Part print with two shaded views. Sizes in mm from the minimum x, y, z corner. A direction names the side the tool comes from. Round coordinates to 2 decimals unless told otherwise and drop trailing zeros. Write each loop counter-clockwise with the first axis right and the second up, starting at its lowest first coordinate (ties: lowest second). Pieces come first, ordered by that corner, then holes. Notation, with made-up numbers: M 74,49 L 110,49 A16 cw 110,74 Z; hole C 47,85.5 d4. An arc over 180 degrees is marked long. Use one line per item in the form item = value. Start each with the question number.
Item 1: Cut at C-C, the plane y = 4.75. Give the cut face in (x, z) (1 decimal).
Item 2: Flat gauge pins, fed straight in: pin 1 Ø1 at (y, z) = (1.5, 16) entering from +X; pin 2 Ø4 at (x, z) = (31.51, 12.7) entering from -Y; pin 3 Ø1.8 at (x, z) = (12.46, 12.7) entering from +Y; pin 4 Ø1.5 at (x, y) = (6, 3) entering from -Z. Where does each tip first touch, or does it go through?
Item 3: Mould opens along Z. For the marked faces 1, 2, 3 and 4 say: +Z half, -Z half, draft (parallel to the pull), parting line (faces both ways), or undercut.
Item 4: Probe L1, parallel to X at y = 4.5, z = 12.7 (1 decimal); L2, parallel to X at y = 3.75, z = 10 (1 decimal); L3, parallel to Y at x = 29, z = 9.5. List the from-to ranges inside material, lowest first.
Item 5: Which spindle directions (+Z, -Z, +X, -X, +Y, -Y) get a long thin tool onto all of the face, cutting with end or side? Do the marked faces 5, 6 and 7. Say none if no direction does.
Item 6: Cut at A-A, the plane z = 12.7. Give the cut face in (x, y) (1 decimal).
Item 7: Cut at B-B, the plane x = 32. Give the cut face in (y, z) (1 decimal), then the cut area to 3 significant figures.
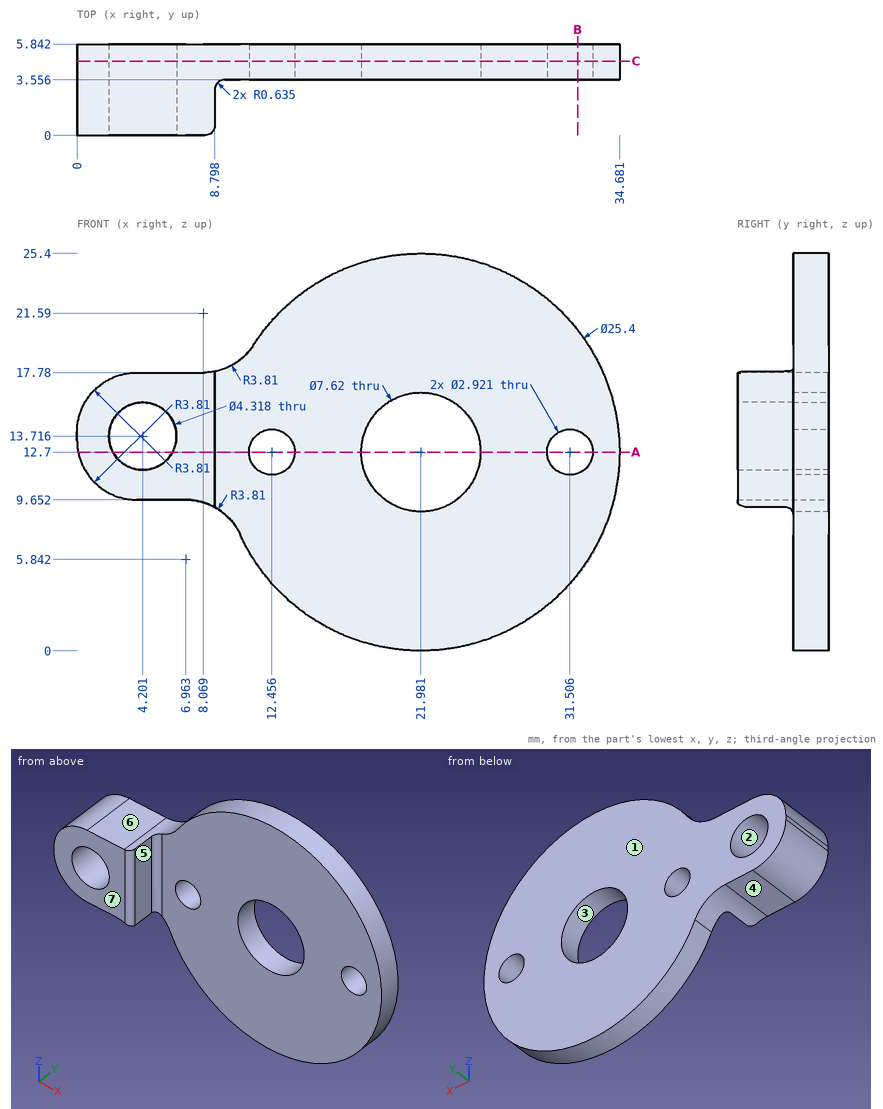
Model answer:
q1.outline = M 0,13.5 A3.8 ccw 3.8,9.7 L 7,9.7 A3.8 cw 10.4,7.4 A12.7 ccw long 11.3,19.5 A3.8 cw 8.1,17.8 L 3.8,17.8 A3.8 ccw 0,14 Z; hole C 4.2,13.7 d4.3; hole C 12.5,12.7 d2.9; hole C 22,12.7 d7.6; hole C 31.5,12.7 d2.9
q2.pin_1 = 8.8
q2.pin_2 = 3.56
q2.pin_3 = through
q2.pin_4 = 9.65
q3.face_1 = draft
q3.face_2 = undercut
q3.face_3 = undercut
q3.face_4 = -Z half
q4.L1 = 0.1 to 2.3, 6.1 to 11, 13.9 to 18.2, 25.8 to 30, 33 to 34.7
q4.L2 = 2.2 to 19.3, 24.7 to 34.4
q4.L3 = 3.56 to 5.84
q5.face_5 = +Z, -Z, +X, -Y
q5.face_6 = +Z, -X, +Y, -Y
q5.face_7 = +Z, -Z, +X, -X, -Y
q6.outline = M 0.1,0 L 2.3,0 L 2.3,5.8 L 0.1,5.8 Z; M 6.1,0 L 8.2,0 A0.6 ccw 8.8,0.6 L 8.8,2.9 A0.6 cw 9.4,3.6 L 11,3.6 L 11,5.8 L 6.1,5.8 Z; M 13.9,3.6 L 18.2,3.6 L 18.2,5.8 L 13.9,5.8 Z; M 25.8,3.6 L 30,3.6 L 30,5.8 L 25.8,5.8 Z; M 33,3.6 L 34.7,3.6 L 34.7,5.8 L 33,5.8 Z
q7.outline = M 3.6,4.9 L 5.8,4.9 L 5.8,11.3 L 3.6,11.3 Z; M 3.6,14.1 L 5.8,14.1 L 5.8,20.5 L 3.6,20.5 Z
q7.area = 29.4 mm²
